Answer from the drawing. Dimensions are ordinates in mm from the lowest x, y and z of the part. A direction names the side the tool comes from. Coordinates: 2 decimals unless noted, no trailing zeros. Loops run counter-clockwise (first coordinate to the right, second up) from the corner with the lowest first, then second, coordinate; pieces in that order, holes last. Notation, with made-up numbers: (0, 70) -> (28, 70) arc R15 cw to (28, 80) -> close; hole circle Ø9 at (-30.5, 54). An arc over 180 degrees is marked (long way). Use a Markdown table: item, result.
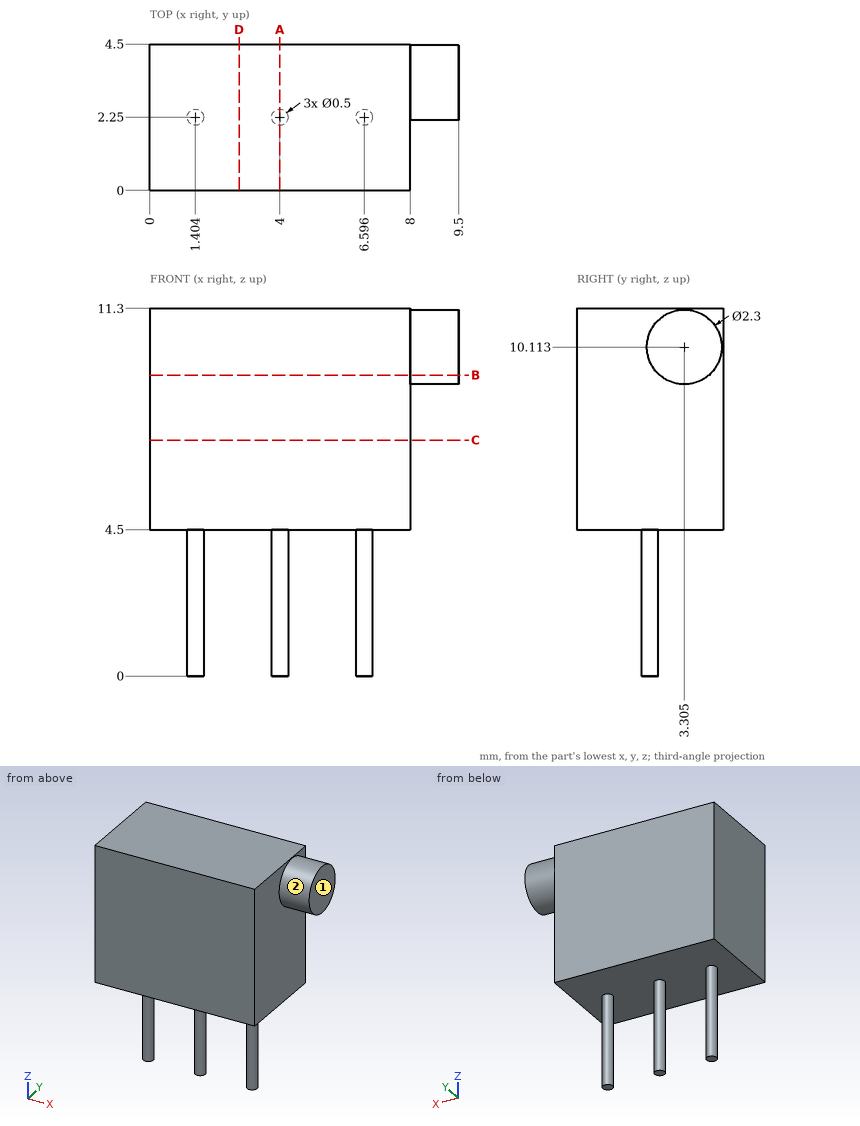
Q1. Section C-C on z = 7.25 is taken. Determine the outline of the cut face in (x, y), and give its area (3 significant figures).
Solved:
| item | result |
|---|---|
| outline | (0, 0) -> (8, 0) -> (8, 4.5) -> (0, 4.5) -> close |
| area | 36.0 mm² |
Q2. For the marked faces 1 and 2, determine the directions among +Z, -Z, +X, -X, +Y, -Y from which every point of the face is accessible in a straight line to the end or side of a thin tool.
Solved:
| item | result |
|---|---|
| face 1 | +Z, -Z, +X, +Y, -Y |
| face 2 | +X |
Q3. Consider line 1 (X direction, y = 3.2, z = 5.25); line 2 (Z direction, x = 1, y = 0.6); line 3 (Z direction, x = 8.5, y = 3.05). Determine where each line is inside the solid, lowest interval first. Write a range as [from, to].
Solved:
| item | result |
|---|---|
| line 1 | [0, 8] |
| line 2 | [4.5, 11.3] |
| line 3 | [8.99, 11.23] |
Q4. Section B-B on z = 9.25 is taken. Determine the outline of the cut face in (x, y) (3 decimals).
Solved:
| item | result |
|---|---|
| outline | (0, 0) -> (8, 0) -> (8, 2.545) -> (9.5, 2.545) -> (9.5, 4.065) -> (8, 4.065) -> (8, 4.5) -> (0, 4.5) -> close |
Q5. Section A-A on x = 4 is taken. Determine the outline of the cut face in (y, z).
Solved:
| item | result |
|---|---|
| outline | (0, 4.5) -> (2, 4.5) -> (2, 0) -> (2.5, 0) -> (2.5, 4.5) -> (4.5, 4.5) -> (4.5, 11.3) -> (0, 11.3) -> close |
Q6. Given pin 1 Ø1 at (x, y) = (6, 0.5) entering from -Z; pin 2 Ø1 at (y, z) = (2, 7) entering from -X; pin 3 Ø3 at (x, z) = (4.5, 1.5) entering from +Y, each flat-ended and moving along its own axis, determine where each tip first touches the part or whether it passes through.
Solved:
| item | result |
|---|---|
| pin 1 | z = 4.5 |
| pin 2 | x = 0 |
| pin 3 | y = 2.5 |
Q7. Section D-D on x = 2.75 is taken. Determine the outline of the cut face in (y, z), and give its area (3 significant figures).
Solved:
| item | result |
|---|---|
| outline | (0, 4.5) -> (4.5, 4.5) -> (4.5, 11.3) -> (0, 11.3) -> close |
| area | 30.6 mm² |
